Input: part model. Units: mm. Frame: model coordinates. Coordinates: 2 decimals unless noted, no trailing zeros. Order: outer loops, then holes, each group sorted by start corner. A loop starts at its lowest first (then second) coordinate and runs counter-clockwise, first axis right, second up. Notation, with made-up numbers: (19, -8.5) - (29, -8.5) arc R6 ccw to (29, -1.5) - close; hole circle Ø6 at (58, 33). An arc over 180 degrees is marked (long way). One line per question, with ' | ' between items.
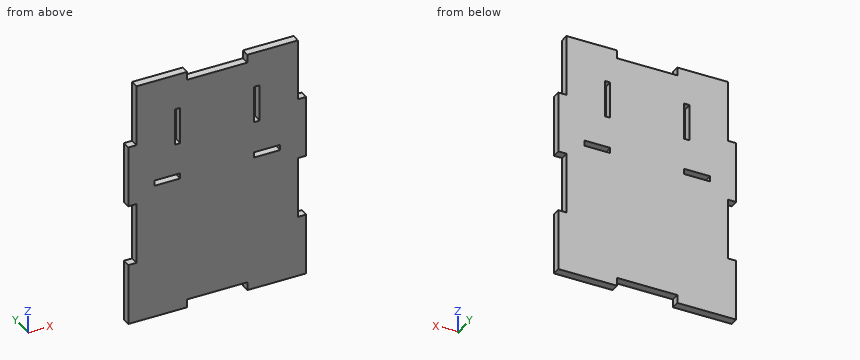
from build123d import *

# Parameters (mm, degrees)
SKETCH1_W           = 130
SKETCH1_H           = 180
BOSS_EXTRUDE1_DEPTH = 6
SKETCH2_W           = 6
SKETCH2_H           = 45
SKETCH2_H_2         = 39
SKETCH2_H_3         = 6
SKETCH2_W_2         = 44
SKETCH2_W_3         = 15
SKETCH2_H_4         = 4
SKETCH2_W_4         = 4
SKETCH2_W_5         = 19
SKETCH2_H_5         = 27
CUT_EXTRUDE1_DEPTH  = 223.117086241


with BuildPart() as part:
    # Sketch1 → Boss-Extrude1 (new body)
    with BuildSketch(Plane(origin=(0, 0, 0), x_dir=(1, 0, 0), z_dir=(0, 1, 0))):
        with Locations((65, 90)):
            Rectangle(SKETCH1_W, SKETCH1_H)
    extrude(amount=BOSS_EXTRUDE1_DEPTH)

    # Sketch2 → Cut-Extrude1 (cut, through all)
    with BuildSketch(Plane(origin=(0, 6, 0), x_dir=(1, 0, 0), z_dir=(0, 1, 0))):
        with Locations((3, 112.5)):
            Rectangle(SKETCH2_W, SKETCH2_H)
        with Locations((3, 25.5)):
            Rectangle(SKETCH2_W, SKETCH2_H_2)
        with Locations((3, 3)):
            Rectangle(SKETCH2_W, SKETCH2_H_3)
        with Locations((127, 22.5)):
            Rectangle(SKETCH2_W, SKETCH2_H)
        with Locations((65, 3)):
            Rectangle(SKETCH2_W_2, SKETCH2_H_3)
        with Locations((127, 112.5)):
            Rectangle(SKETCH2_W, SKETCH2_H)
        with Locations((103.5, 78)):
            Rectangle(SKETCH2_W_3, SKETCH2_H_4)
        with Locations((94, 78)):
            Rectangle(SKETCH2_W_4, SKETCH2_H_4)
        with Locations((28.5, 78)):
            Rectangle(SKETCH2_W_5, SKETCH2_H_4)
        with Locations((36, 39.5)):
            Rectangle(SKETCH2_W_4, SKETCH2_H_5)
        with Locations((94, 39.5)):
            Rectangle(SKETCH2_W_4, SKETCH2_H_5)
        with Locations((65, 177)):
            Rectangle(SKETCH2_W_2, SKETCH2_H_3)
    extrude(amount=-CUT_EXTRUDE1_DEPTH, mode=Mode.SUBTRACT)


solid = part.part
Item 1: Section A-A on y = 1.3. Count the separate pieces of the cut face and the enclosed holes in it, and give its area (3 significant figures).
Data:
separate pieces: 1 | enclosed holes: 4 | area: 21,400 mm^2
Item 2: Section B-B on z = -94.5. Return the cut outline in (x, y).
Data:
outline: (6, 0) - (124, 0) - (124, 6) - (6, 6) - close
Item 3: Ray query, line 1 (X direction, y = 4.7, z = -28.5); line 2 (Z direction, x = 28.5, y = 2.3); line 3 (X direction, y = 2.45, z = -119). Return the intervals inside material, ascending.
Data:
line 1: 6 to 34, 38 to 92, 96 to 124 | line 2: -180 to -80, -76 to 0 | line 3: 6 to 124
Item 4: Contact query for flat-ended pins moving along their axis: P1, Ø3, axis at y = 2, z = -35, coming from the +X side; P2, Ø3, axis at y = 2.5, z = -33.5, coming from the -X side. Output: stop coordinate, or through.
Data:
P1: x = 124 | P2: x = 6
Item 5: Section C-C on x = 53.5. Return the cut outline in (y, z), and give its area (3 significant figures).
Data:
outline: (0, -174) - (6, -174) - (6, -6) - (0, -6) - close | area: 1,010 mm^2
